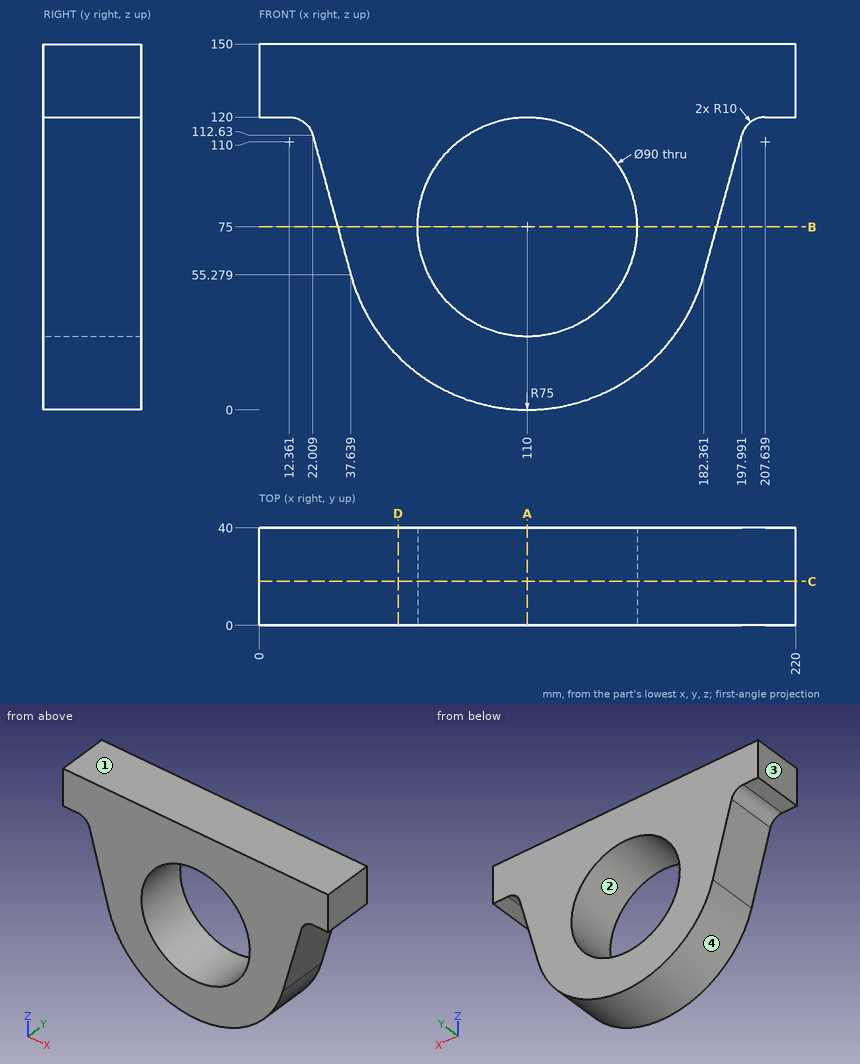
Job drawing, mm, ordinate dimensions from the low corner. One solid piece. Round coordinates to 2 decimals unless told otherwise and drop trailing zeros. Order: outer loops, then holes, each group sorted by start corner. A loop starts at its lowest first (then second) coordinate and runs counter-clockwise, first axis right, second up. Notation, with made-up numbers: (19, 61) -> (46, 61) arc R17 cw to (46, 73) -> close; hole circle Ø8 at (85, 37). An arc over 180 degrees is marked (long way). Write item = value, one per line.
(1) Flat gauge pins, fed straight in: P1, Ø3.5, axis at x = 212, y = 18.5, coming from the -Z side; P2, Ø3, axis at y = 16.5, z = 94.5, coming from the -X side; P3, Ø1.5, axis at y = 27, z = 117, coming from the -X side; P4, Ø5, axis at x = 133.5, z = 36.5, coming from the -Y side. Where does each tip first touch, or does it go through?
Answers follow:
P1 = 120
P2 = 26.54
P3 = 18.68
P4 = 0
(2) Cut at D-D (x = 57). Write the cut outline in (y, z).
Answers follow:
outline = (0, 21.93) -> (40, 21.93) -> (40, 150) -> (0, 150) -> close
(3) Drill centre lines: L1, parallel to X at y = 16, z = 75 (1 decimal); L2, parallel to Z at x = 93, y = 25 (1 decimal); L3, parallel to Z at x = 73.5, y = 28.5. Where is each one in solid material? Low to high.
Answers follow:
L1 = 32.3 to 65, 155 to 187.7
L2 = 2 to 33.3, 116.7 to 150
L3 = 9.48 to 48.68, 101.32 to 150
(4) Cut at C-C (y = 18). Write the cut outline in (x, z), plus the area to 3 significant figures.
Answers follow:
outline = (0, 120) -> (12.36, 120) arc R10 cw to (22.01, 112.63) -> (37.64, 55.28) arc R75 ccw to (182.36, 55.28) -> (197.99, 112.63) arc R10 cw to (207.64, 120) -> (220, 120) -> (220, 150) -> (0, 150) -> close; hole circle Ø90 at (110, 75)
area = 16,700 mm²
(5) Pull direction X, two halves, no side cores. Call the marked faces 1, 2, 3 and 4: +X half, -X half, draft (parallel to the pull), parting line (faces both ways), or undercut.
Answers follow:
face_1 = draft
face_2 = undercut
face_3 = -X half
face_4 = parting line
(6) Cut at B-B (z = 75). Write the cut outline in (x, y) (1 decimal), plus the area to 3 significant figures.
Answers follow:
outline = (32.3, 0) -> (65, 0) -> (65, 40) -> (32.3, 40) -> close; (155, 0) -> (187.7, 0) -> (187.7, 40) -> (155, 40) -> close
area = 2,620 mm²
(7) Cut at A-A (x = 110). Write the cut outline in (y, z), plus the area to 3 significant figures.
Answers follow:
outline = (0, 0) -> (40, 0) -> (40, 30) -> (0, 30) -> close; (0, 120) -> (40, 120) -> (40, 150) -> (0, 150) -> close
area = 2,400 mm²
